Answer from the drawing. Dimensions are ordinates in mm from the lowest x, y and z of the part. A direction names the side the tool comes from. Give positions to 0.01 mm unless a question says otherwise; leave off trailing zeros. Order: outer loops, then holes, each group sorted by start corner. A loop starts at its lowest first (then second) coordinate and runs counter-clockwise, first axis right, second up. Notation, with made-up numbers: (39, -23) - (72, -23) arc R31 ccw to (72, 12) - close; hole circle Ø1 at (18, -14.5). An arc over 180 degrees is marked (long way). Write each question's results on one line, items separated by ' | '.
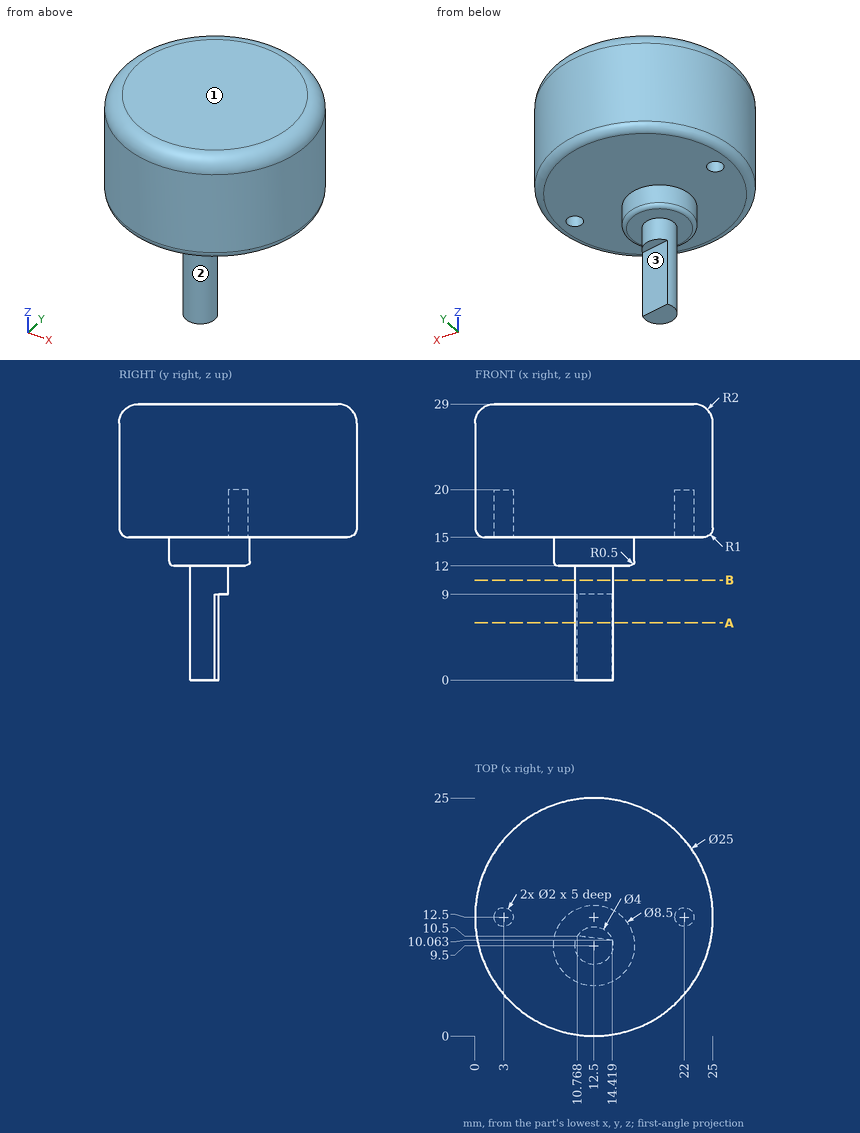
1. A tool of negligible diameter and unlimited length cuts with its end or side. For the marked faces 1, 2 and 3, from which of +Z, -Z, +X, -X, +Y, -Y can it reach the whole face along a straight path? Write none if from no direction.
Answer list:
face 1: +Z, +X, -X, +Y, -Y | face 2: -Z | face 3: -Z, +X, +Y
2. Straight lines are drawn through the part: line 1 (Z direction, x = 4.25, y = 8.5); line 2 (Z direction, x = 15, y = 12); line 3 (Y direction, x = 22, z = 17.5) (1 decimal). For each, find the intervals that lie inside material, in ascending order. Write a range as [from, to].
Answer list:
line 1: [15, 29] | line 2: [12, 29] | line 3: [4.4, 11.5], [13.5, 20.6]
3. A cutting plane is placed at B-B, the plane z = 10.5. Write down the section's boundary in (x, y), then the cut area to 3 significant figures.
Answer list:
outline: circle Ø4 at (12.5, 9.5) | area: 12.6 mm^2
4. Given P1, Ø2, axis at x = 3.5, y = 12.5, coming from the -Z side; P2, Ø2, axis at y = 14.5, z = 20, coming from the -X side; P3, Ø3, axis at x = 3.5, z = 20.5, coming from the -Y side, each flat-ended and moving along its own axis, determine where each tip first touches the part or whether it passes through.
Answer list:
P1: z = 15 | P2: x = 0.04 | P3: y = 2.5
5. A cutting plane is placed at A-A, the plane z = 6. Write down the section's boundary in (x, y).
Answer list:
outline: (10.77, 10.5) arc R2 ccw (long way) to (14.42, 10.06) - close
